Input: part model. Units: mm. Frame: model coordinates. A direction names the side the tool comes from. Coordinates: 2 decimals unless noted, no trailing zeros. Write each loop counter-clockwise with the first axis right and the second up, starting at its lowest first coordinate (ties: lowest second). Pieces come first, ordered by that corner, then holes.
1) Line query: L1, parallel to Y at x = -4.5, z = 7.75; L2, parallel to Y at x = 4.5, z = 13.1; L3, parallel to Y at x = 0, z = 6.8. Output: solid intervals per line, ascending.
2) Section query B-B (y = -30.5). Output: boundary loops of the cut face in (x, z).
3) Pin query (flat end, axial travel): pin 1 Ø3 at (x, y) = (-4.5, -49) entering from +Z; pin 2 Ø5 at (x, z) = (-42, 5) entering from -Y; pin 3 Ø4.5 at (x, y) = (3.5, -50) entering from +Z; pin 4 Ø8 at (x, y) = (-4.5, -35.5) entering from +Z. Return the tip coordinate at first contact, or that it passes through.
4) Section query A-A (z = 13). Output: boundary loops of the cut face in (x, y).
5) Section query C-C (z = 4). State how many separate pieces and enclosed holes the cut face has, then the cut area to 3 significant figures.
6) Section query D-D (x = 19). Output: boundary loops of the cut face in (y, z), then the cut area to 3 significant figures.
7) Set-up query: faces 5 (the cylindrical face through (-7.89, -54.1, 11.45)), 6 (the cylindrical face through (3.715, -76.242, 5.465)), 7 (the cylindrical face through (7.89, -43.9, 11.45)), 8 (the flat face through (0, -55, 12)). Return all of +Z, -Z, +X, -X, +Y, -Y with unobstructed straight access to the full face (end or side cutting, diameter ignored); none if empty.
8) Draft query along X for faces 1 (the flat face through (-4, -32, 8)), 2 (the flat face through (-8.75, -48, 6)), 3 (the cylindrical face through (4.04, -51.05, 12.54)), 4 (the cylindrical face through (42.15, -4.54, 3.37)). Return one class per face: pulls with the +X half, pulls with the -X half, needs draft (parallel to the pull), parting line crosses it, or undercut.
from build123d import *

# Parameters (mm, degrees)
SKETCH3_R           = 8.05
BOSS_EXTRUDE1_DEPTH = 8
SKETCH4_R           = 8.05
SKETCH4_R_2         = 4.3
BOSS_EXTRUDE2_DEPTH = 3
CHAMFER1_SIZE       = 3
FILLET1_R           = 11
SKETCH5_R           = 1.65
CUT_EXTRUDE1_DEPTH  = 85.020655349
SKETCH6_R           = 3
CUT_EXTRUDE2_DEPTH  = 3
SKETCH7_R           = 2.1
CUT_EXTRUDE3_DEPTH  = 5
SKETCH8_R           = 1.65
CUT_EXTRUDE4_DEPTH  = 93.528214752
CUT_EXTRUDE5_DEPTH  = 93.528214752
FILLET2_R           = 5
FILLET3_R           = 2
BOSS_EXTRUDE3_START = 7
SKETCH10_W          = 17.5
SKETCH10_H          = 12
SKETCH10_R          = 2.1
BOSS_EXTRUDE3_DEPTH = 7
FILLET4_R           = 3
BOSS_EXTRUDE4_START = 7
SKETCH11_R          = 2.1
SKETCH11_R_2        = 1.65
BOSS_EXTRUDE4_DEPTH = 7


with BuildPart() as part:
    # Sketch3 → Boss-Extrude1 (new body)
    with BuildSketch(Plane.XY):
        with BuildLine():
            Line((-31.937438845, -2), (-45.623026261, -2))
            Line((-45.623026261, -2), (-45.623026261, -10))
            Line((-45.623026261, -10), (-35.623026261, -10))
            ThreePointArc((-35.623026261, -10), (-26.529067588, -25.791637654), (-11, -35.327043465))
            Line((-11, -35.327043465), (-11, -80.1))
            Line((-11, -80.1), (11, -80.1))
            Line((11, -80.1), (11, -35.327043465))
            ThreePointArc((11, -35.327043465), (26.529067588, -25.791637654), (35.623026261, -10))
            Line((35.623026261, -10), (45.623026261, -10))
            Line((45.623026261, -10), (45.623026261, -2))
            Line((45.623026261, -2), (31.937438845, -2))
            ThreePointArc((31.937438845, -2), (0, -32), (-31.937438845, -2))
        make_face()
        with Locations((0, -69.1)):
            Circle(SKETCH3_R, mode=Mode.SUBTRACT)
    extrude(amount=BOSS_EXTRUDE1_DEPTH)

    # Sketch4 → Boss-Extrude2 (add)
    with BuildSketch(Plane.XY):
        with Locations(Location((0, -69.1, 0), (0, 0, 180))):
            Circle(SKETCH4_R)
        with Locations(Location((0, -69.1, 0), (0, 0, 180))):
            Circle(SKETCH4_R_2, mode=Mode.SUBTRACT)
    extrude(amount=BOSS_EXTRUDE2_DEPTH)

    # Chamfer1
    chamfer1_edges = [part.edges().sort_by_distance(p)[0] for p in [
        (0, -80.1, 0),
    ]]
    chamfer(chamfer1_edges, length=CHAMFER1_SIZE)

    # Fillet1
    fillet1_edges = [part.edges().sort_by_distance(p)[0] for p in [
        (-11, -80.1, 5.5),
        (11, -80.1, 5.5),
    ]]
    fillet(fillet1_edges, radius=FILLET1_R - 0.0001)  # a hair under: the kernel refuses the full size

    # Sketch5 → Cut-Extrude1 (cut, through all)
    with BuildSketch(Plane.XZ.offset(10)):
        with Locations((40.623026261, 4)):
            Circle(SKETCH5_R)
    cut_extrude1 = extrude(amount=-CUT_EXTRUDE1_DEPTH, mode=Mode.SUBTRACT)

    # Sketch6 → Cut-Extrude2 (cut)
    with BuildSketch(Plane.XZ.offset(10)):
        with Locations((40.623026261, 4)):
            Circle(SKETCH6_R)
    cut_extrude2 = extrude(amount=-CUT_EXTRUDE2_DEPTH, mode=Mode.SUBTRACT)

    # Mirror1: Cut-Extrude1, Cut-Extrude2 across plane
    add(cut_extrude1.mirror(Plane(origin=(0, 0, 0), x_dir=(0, 0, 1), z_dir=(1, 0, 0))), mode=Mode.SUBTRACT)
    add(cut_extrude2.mirror(Plane(origin=(0, 0, 0), x_dir=(0, 0, 1), z_dir=(1, 0, 0))), mode=Mode.SUBTRACT)

    # Sketch7 → Cut-Extrude3 (cut)
    with BuildSketch(Plane.XY.offset(8)):
        with Locations((-4.5, -49)):
            Circle(SKETCH7_R)
        with Locations((4.5, -49)):
            Circle(SKETCH7_R)
    extrude(amount=-CUT_EXTRUDE3_DEPTH, mode=Mode.SUBTRACT)

    # Sketch8 → Cut-Extrude4 (cut, through all)
    with BuildSketch(Plane.XY.offset(8)):
        with Locations((4.5, -49)):
            Circle(SKETCH8_R)
        with Locations((-4.5, -49)):
            Circle(SKETCH8_R)
    extrude(amount=-CUT_EXTRUDE4_DEPTH, mode=Mode.SUBTRACT)

    # Sketch9 → Cut-Extrude5 (cut, through all)
    with BuildSketch(Plane.XY.offset(8)):
        with BuildLine():
            Line((-8.75, -35.950486784), (-8.75, -57.333854187))
            ThreePointArc((-8.75, -57.333854187), (-10.422331793, -60.48218818), (-11, -64))
            Line((-11, -64), (-11, -35.327043465))
            ThreePointArc((-11, -35.327043465), (-9.879918795, -35.656517001), (-8.75, -35.950486784))
        make_face()
        with BuildLine():
            Line((8.75, -57.333854187), (8.75, -35.950486784))
            ThreePointArc((8.75, -35.950486784), (9.879918795, -35.656517001), (11, -35.327043465))
            Line((11, -35.327043465), (11, -64))
            ThreePointArc((11, -64), (10.422331793, -60.48218818), (8.75, -57.333854187))
        make_face()
    extrude(amount=-CUT_EXTRUDE5_DEPTH, mode=Mode.SUBTRACT)

    # Fillet2
    fillet2_edges = [part.edges().sort_by_distance(p)[0] for p in [
        (-8.75, -35.950486784, 4),
        (-8.75, -57.333854187, 4),
        (8.75, -57.333854187, 4),
        (8.75, -35.950486784, 4),
    ]]
    fillet(fillet2_edges, radius=FILLET2_R)

    # Fillet3
    fillet3_edges = [part.edges().sort_by_distance(p)[0] for p in [
        (-45.623026261, -2, 4),
        (-31.937438845, -2, 4),
        (31.937438845, -2, 4),
        (45.623026261, -2, 4),
        (45.623026261, -10, 4),
        (35.623026261, -10, 4),
        (-35.623026261, -10, 4),
        (-45.623026261, -10, 4),
    ]]
    fillet(fillet3_edges, radius=FILLET3_R - 0.0001)  # a hair under: the kernel refuses the full size

    # Sketch10 → Boss-Extrude3 (add)
    with BuildSketch(Plane.XY.offset(8).offset(BOSS_EXTRUDE3_START)):
        with Locations((0, -49)):
            Rectangle(SKETCH10_W, SKETCH10_H)
        with Locations((4.5, -49)):
            Circle(SKETCH10_R, mode=Mode.SUBTRACT)
        with Locations((-4.5, -49)):
            Circle(SKETCH10_R, mode=Mode.SUBTRACT)
    extrude(amount=-BOSS_EXTRUDE3_DEPTH)

    # Fillet4
    fillet4_edges = [part.edges().sort_by_distance(p)[0] for p in [
        (-8.75, -43, 11.5),
        (-8.75, -55, 11.5),
        (8.75, -55, 11.5),
        (8.75, -43, 11.5),
    ]]
    fillet(fillet4_edges, radius=FILLET4_R)

    # Sketch11 → Boss-Extrude4 (add)
    # profile 1 of 2: a face of its own
    with BuildSketch(Plane.XY.offset(3).offset(BOSS_EXTRUDE4_START)):
        with Locations((4.5, -49)):
            Circle(SKETCH11_R)
        with Locations((4.5, -49)):
            Circle(SKETCH11_R_2, mode=Mode.SUBTRACT)
    # profile 2 of 2: a face of its own
    with BuildSketch(Plane.XY.offset(3).offset(BOSS_EXTRUDE4_START)):
        with Locations((-4.5, -49)):
            Circle(SKETCH11_R)
        with Locations((-4.5, -49)):
            Circle(SKETCH11_R_2, mode=Mode.SUBTRACT)
    extrude(amount=-BOSS_EXTRUDE4_DEPTH)


solid = part.part
Answer:
1. L1: y = -79.14 to -75.77, -62.43 to -50.65, -47.35 to -31.68
1. L2: y = -55 to -51.1, -46.9 to -43
1. L3: y = -80.1 to -77.15, -61.05 to -32
2. outline: (-20.95, 0) - (-9.68, 0) - (-9.68, 8) - (-20.95, 8) - close; (9.68, 0) - (20.95, 0) - (20.95, 8) - (9.68, 8) - close
3. pin 1: passes through
3. pin 2: stops at y = -10
3. pin 3: stops at z = 15
3. pin 4: stops at z = 8
4. outline: (-8.75, -52) arc R3 ccw to (-5.75, -55) - (5.75, -55) arc R3 ccw to (8.75, -52) - (8.75, -46) arc R3 ccw to (5.75, -43) - (-5.75, -43) arc R3 ccw to (-8.75, -46) - close; hole circle Ø4.2 at (-4.5, -49); hole circle Ø4.2 at (4.5, -49)
5. separate pieces: 3
5. enclosed holes: 3
5. area: 1,180 mm2
6. outline: (-31.75, 0) - (-25.75, 0) - (-25.75, 8) - (-31.75, 8) - close
6. area: 48.0 mm2
7. face 5: +Z, -X, -Y
7. face 6: +Z
7. face 7: +Z, +X, +Y
7. face 8: +Z, +X, -X, -Y
8. face 1: needs draft
8. face 2: pulls with the -X half
8. face 3: undercut
8. face 4: undercut
